from build123d import *

# Parameters (mm, degrees)
SKETCH1_R                      = 15
EXTRUDE1_DEPTH                 = 10
EXTRUDE3_DEPTH                 = 10
CIRPATTERN1_COUNT              = 20
F_8_2_8_2_DIAMETER_HOLE1_D     = 8.2
F_8_2_8_2_DIAMETER_HOLE1_DEPTH = 10
F_8_2_8_2_DIAMETER_HOLE1_TIP   = 2.463528538
SKETCH4_W                      = 24
SKETCH4_H                      = 9.5
EXTRUDE4_DEPTH                 = 4.6
F_1_5_1_5_DIAMETER_HOLE1_D     = 1.5
F_1_5_1_5_DIAMETER_HOLE1_DEPTH = 150
F_1_5_1_5_DIAMETER_HOLE1_TIP   = 0.450645464
EXTRUDE5_DEPTH                 = 6


with BuildPart() as part:
    # Sketch1 → Extrude1 (new body)
    with BuildSketch(Plane.XY):
        Circle(SKETCH1_R)
    extrude(amount=EXTRUDE1_DEPTH)

    # Sketch2 → Extrude3 (add)
    with BuildSketch(Plane.XY.offset(10)):
        Polygon((1.4, 14.704480908), (1, 16.404480908), (-1, 16.404480908), (-1.4, 14.704480908), align=None)
    extrude3 = extrude(amount=-EXTRUDE3_DEPTH)

    # CirPattern1: Extrude3 ×20 about axis
    cirpattern1_axis = Axis((0, 0, 0), (0, 0, 1))
    for i in range(1, CIRPATTERN1_COUNT):
        add(extrude3.rotate(cirpattern1_axis, i * 360 / CIRPATTERN1_COUNT))

    # Ø8.2 (8.2) Diameter Hole1
    with Locations(Plane(origin=(0, 0, 0), x_dir=(-1, 0, 0), z_dir=(0, 0, -1))):
        with Locations((0, 0)):
            Hole(F_8_2_8_2_DIAMETER_HOLE1_D / 2, depth=F_8_2_8_2_DIAMETER_HOLE1_DEPTH)
            with Locations((0, 0, -(F_8_2_8_2_DIAMETER_HOLE1_DEPTH + F_8_2_8_2_DIAMETER_HOLE1_TIP / 2))):  # 118° drill point
                Cone(0, F_8_2_8_2_DIAMETER_HOLE1_D / 2, F_8_2_8_2_DIAMETER_HOLE1_TIP, mode=Mode.SUBTRACT)

    # Sketch4 → Extrude4 (cut)
    with BuildSketch(Plane.XY.offset(10)):
        Rectangle(SKETCH4_W, SKETCH4_H)
    extrude(amount=-EXTRUDE4_DEPTH, mode=Mode.SUBTRACT)

    # Ø1.5 (1.5) Diameter Hole1
    with Locations(Plane(origin=(10, 0, 0), x_dir=(-1, 0, 0), z_dir=(0, 0, -1))):
        with Locations((0, 0), (20, 0)):
            Hole(F_1_5_1_5_DIAMETER_HOLE1_D / 2, depth=F_1_5_1_5_DIAMETER_HOLE1_DEPTH)
            with Locations((0, 0, -(F_1_5_1_5_DIAMETER_HOLE1_DEPTH + F_1_5_1_5_DIAMETER_HOLE1_TIP / 2))):  # 118° drill point
                Cone(0, F_1_5_1_5_DIAMETER_HOLE1_D / 2, F_1_5_1_5_DIAMETER_HOLE1_TIP, mode=Mode.SUBTRACT)

    # Sketch6 → Extrude5 (cut)
    with BuildSketch(Plane.XY.offset(10)):
        Polygon((3.908986866, 6.743131445), (-3.885229699, 6.756847651), (-7.794216565, 0.013716207), (-3.908986866, -6.743131445), (3.885229699, -6.756847651), (7.794216565, -0.013716207), align=None)
    extrude(amount=-EXTRUDE5_DEPTH, mode=Mode.SUBTRACT)


solid = part.part
Model file for the job. Use its own axes, mm. A direction names the side the tool comes from. Give positions to 0.01 mm unless a question says otherwise; leave off trailing zeros. Write each loop counter-clockwise with the first axis right and the second up, starting at its lowest first coordinate (ties: lowest second). Pieces come first, ordered by that corner, then holes. Notation, with made-up numbers: (-29.5, 38) - (11.5, 38) arc R23 ccw to (11.5, 53) - close; hole circle Ø3 at (6, -28.5). An arc over 180 degrees is marked (long way). Answer as CSV lines item,"result".
1. Drill centre lines: L1, parallel to Y at x = 10, z = 4.3; L2, parallel to X at y = -13.5, z = 5; L3, parallel to Y at x = -0.5, z = 6. Where is each one in solid material? Low to high. Write a range as [from, to].
Responses:
L1,"y = [-13.01, -11.61], [-11.18, -0.75], [0.75, 11.18], [11.61, 13.01]"
L2,"x = [-9.33, -8.42], [-6.54, 6.54], [8.42, 9.33]"
L3,"y = [-16.4, -6.75], [6.75, 16.4]"
2. 3-axis set-ups, long thin cutter, end or side, ignore diameter. For faces 4 (the face through (-14.813, 2.36, 4.93)), 5 (the face through (5.08, 15.6, 5.07)), 6 (the face through (1.17, -15.68, 5.07)): which of +Z, -Z, +X, -X, +Y, -Y reach the whole face in a straight line?
Responses:
face 4,"+Z, -Z, -X"
face 5,"+Z, -Z, +X, +Y"
face 6,"+Z, -Z, -Y"
3. Two-plate mould, pull along X, no slides. Class faces 1 (the face through (-15.258, -3.723, 5.07)), 2 (the face through (15.258, 3.723, 5.07)), 3 (the face through (8.3, 13.4, 5.1)): +X half, -X half, draft (parallel to the pull), parting line (faces both ways), or undercut.
Responses:
face 1,"-X half"
face 2,"+X half"
face 3,"undercut"
4. Band-saw the part on C-C (z = 3). Count the separate pieces of the cut face and the enclosed holes in it, and give its area (3 significant figures).
Responses:
separate pieces,"1"
enclosed holes,"3"
area,"717 mm2"
5. Pin check, flat tips, straight feed: pin 1 (3.5 mm diameter, centred on x = -9.5, y = -1.5, fed in from +Z); pin 2 (11 mm diameter, centred on x = 4, y = 3.5, fed in from +Z); pin 3 (1.5 mm diameter, centred on y = -12.5, z = 7.5, fed in from -X); pin 4 (3 mm diameter, centred on y = -12.5, z = 2, fed in from +X). Stop position of each tip, or through.
Responses:
pin 1,"stops at z = 5.4"
pin 2,"stops at z = 10"
pin 3,"stops at x = -10.45"
pin 4,"stops at x = 10.45"
6. Band-saw the part on A-A (x = 0). Write the cut outline in (y, z).
Responses:
outline,"(-16.4, 0) - (-4.1, 0) - (-4.1, 4) - (-6.75, 4) - (-6.75, 10) - (-16.4, 10) - close; (4.1, 0) - (16.4, 0) - (16.4, 10) - (6.75, 10) - (6.75, 4) - (4.1, 4) - close"
7. Band-saw the part on B-B (y = -2). Write the cut outline in (x, z).
Responses:
outline,"(-14.87, 0) - (-3.58, 0) - (-3.58, 4) - (-6.64, 4) - (-6.64, 5.4) - (-12, 5.4) - (-12, 10) - (-14.87, 10) - close; (3.58, 0) - (14.87, 0) - (14.87, 10) - (12, 10) - (12, 5.4) - (6.64, 5.4) - (6.64, 4) - (3.58, 4) - close"
